from build123d import *

# Parameters (mm, degrees)
F0_W         = 50.8
F0_H         = 50.8
F16_DEPTH    = 0.635
F13_E4_W     = 50.8
F13_E4_H     = 25.4
F17_DEPTH    = 2.54
F11_E6_W     = 50.8
F11_E6_H     = 25.4
F11_E5_W     = 50.8
F11_E5_H     = 25.4
F18_DEPTH    = 2.54
F9_E0_W      = 25.4
F9_E0_H      = 25.4
F9_E3_W      = 25.4
F9_E3_H      = 25.4
F19_DEPTH    = 2.54
F7_E7_W      = 50.8
F7_E7_H      = 25.4
F20_DEPTH    = 2.54
F3_E1_W      = 50.8
F3_E1_H      = 25.4
F21_DEPTH    = 2.54
F1_E2_W      = 50.8
F1_E2_H      = 25.4
F22_DEPTH    = 2.54
F23_R        = 5.08
F24_T1_DEPTH = 51.7877054869


# Not quite as in the source:
# - a fillet or chamfer that OpenCascade refuses, or shapes differently, is made with other operations: its cross-section is extruded or revolved along the edge and cut away or added
# - the program builds the solid bodies; features that only make, move or delete a surface that nothing else refers to are left out


with BuildPart() as f16:
    # F0 (on Top) → F16 (new body)
    with BuildSketch(Plane.XY):
        Polygon((-25.4, 0), (0, 0), (25.4, 0), (25.4, 50.8), (-25.4, 50.8), align=None)
        Polygon((25.4, 0), (0, 0), (-25.4, 0), (-25.4, -50.8), (25.4, -50.8), align=None)
        with Locations((50.8, -25.4)):
            Rectangle(F0_W, F0_H)
        with Locations((50.8, 25.4)):
            Rectangle(F0_W, F0_H)
        with Locations((-50.8, -25.4)):
            Rectangle(F0_W, F0_H)
        with Locations((-50.8, 25.4)):
            Rectangle(F0_W, F0_H)
    extrude(amount=-F16_DEPTH)

    # F13_E4 (on explicit) → F17 (join, symmetric)
    with BuildSketch(Plane(origin=(-25.4, 0, 0), x_dir=(-1, 0, 0), z_dir=(0, 1, 0))):
        with Locations((25.4, 12.7)):
            Rectangle(F13_E4_W, F13_E4_H)
    extrude(amount=F17_DEPTH, both=True)

    # F11_E6 (on explicit) + F11_E5 (on explicit) → F18 (join, symmetric)
    with BuildSketch(Plane.YZ.offset(-25.4)):
        with Locations((25.4, 12.7)):
            Rectangle(F11_E6_W, F11_E6_H)
    with BuildSketch(Plane(origin=(-25.4, 0, 0), x_dir=(0, -1, 0), z_dir=(-1, 0, 0))):
        with Locations((25.4, 12.7)):
            Rectangle(F11_E5_W, F11_E5_H)
    extrude(amount=F18_DEPTH, both=True, dir=(1, 0, 0))

    # F9_E0 (on explicit) + F9_E3 (on explicit) → F19 (join, symmetric)
    with BuildSketch(Plane.XZ):
        with Locations((12.7, 12.7)):
            Rectangle(F9_E0_W, F9_E0_H)
    with BuildSketch(Plane(origin=(0, 0, 0), x_dir=(-1, 0, 0), z_dir=(0, 1, 0))):
        with Locations((12.7, 12.7)):
            Rectangle(F9_E3_W, F9_E3_H)
    extrude(amount=F19_DEPTH, both=True, dir=(0, -1, 0))

    # F7_E7 (on explicit) → F20 (join, symmetric)
    with BuildSketch(Plane.YZ.offset(25.4)):
        with Locations((25.4, 12.7)):
            Rectangle(F7_E7_W, F7_E7_H)
    extrude(amount=F20_DEPTH, both=True)

    # F3_E1 (on explicit) → F21 (join, symmetric)
    with BuildSketch(Plane(origin=(25.4, 0, 0), x_dir=(0, -1, 0), z_dir=(-1, 0, 0))):
        with Locations((25.4, 12.7)):
            Rectangle(F3_E1_W, F3_E1_H)
    extrude(amount=F21_DEPTH, both=True)

    # F1_E2 (on explicit) → F22 (join, symmetric)
    with BuildSketch(Plane(origin=(25.4, 0, 0), x_dir=(1, 0, 0), z_dir=(0, -1, 0))):
        with Locations((25.4, 12.7)):
            Rectangle(F1_E2_W, F1_E2_H)
    extrude(amount=F22_DEPTH, both=True)

    # F23
    f23_edges = [f16.edges().sort_by_distance(p)[0] for p in [
        (76.2, 0, -0.635),
    ]]
    fillet(f23_edges, radius=F23_R)

    # F24: fillet of radius 5.08 on 1 edges, made by hand

    # F24_s2 → F24_t1 (cut)
    with BuildSketch(Plane.YZ.offset(27.94)):
        with BuildLine():
            ThreePointArc((-50.8, -0.635), (-49.6106555752, -0.1613111503), (-48.3406555752, 0))
            Line((-48.3406555752, 0), (-50.8, 0))
            Line((-50.8, 0), (-50.8, -0.635))
        make_face()
    extrude(amount=F24_T1_DEPTH, mode=Mode.SUBTRACT)


solid = f16.part
Build history of the part. All positions in model axes, mm. A direction names the side the tool comes from. Give positions to 0.01 mm unless a question says otherwise; leave off trailing zeros. Loops run counter-clockwise (first coordinate to the right, second up) from the corner with the lowest first, then second, coordinate; pieces in that order, holes last. Notation, with made-up numbers: (20.5, 36.5) -> (38.5, 36.5) arc R32 cw to (38.5, 72.5) -> close; hole circle Ø7 at (75.25, -3). An arc over 180 degrees is marked (long way). Answer in a Markdown table with one row per item.
Item 1: Slice it at C-C on y = -29.5. Write the cut outline in (x, z) (3 decimals), plus the area to 3 significant figures.
Findings below:
| item | result |
|---|---|
| outline | (-76.2, -0.635) -> (71.12, -0.635) arc R5.08 ccw to (73.579, 0) -> (27.94, 0) -> (27.94, 25.4) -> (22.86, 25.4) -> (22.86, 0) -> (-22.86, 0) -> (-22.86, 25.4) -> (-27.94, 25.4) -> (-27.94, 0) -> (-76.2, 0) -> close |
| area | 353 mm² |
Item 2: Probe line 1 along X through (y, z) = (-25, 7.5); line 2 along Z through (x, y) = (29, 29.5) (3 decimals); line 3 along Y through (x, z) = (-67.5, 11.5). List the from-to ranges inside material, lowest first. Write a range as [from, to].
Findings below:
| item | result |
|---|---|
| line 1 | x = [-27.94, -22.86], [22.86, 27.94] |
| line 2 | z = [-0.635, 0] |
| line 3 | y = [-2.54, 2.54] |
Item 3: Flat gauge pins, fed straight in: P1, Ø3, axis at x = 5, z = 16.5, coming from the +Y side; P2, Ø4, axis at x = -10.5, z = 14.5, coming from the -Y side; P3, Ø8, axis at y = -33.5, z = 6.5, coming from the +X side. Where does each tip first touch, or does it go through?
Findings below:
| item | result |
|---|---|
| P1 | stops at y = 2.54 |
| P2 | stops at y = -2.54 |
| P3 | stops at x = 27.94 |
Item 4: Slice it at D-D on x = -16.5. Write the cut outline in (y, z) (3 decimals).
Findings below:
| item | result |
|---|---|
| outline | (-50.8, -0.635) -> (50.8, -0.635) -> (50.8, 0) -> (2.54, 0) -> (2.54, 25.4) -> (-2.54, 25.4) -> (-2.54, 0) -> (-50.8, 0) -> close |
Item 5: Slice it at A-A on x = 31.5. Write the cut outline in (y, z) (3 decimals).
Findings below:
| item | result |
|---|---|
| outline | (-50.8, -0.635) -> (50.8, -0.635) -> (50.8, 0) -> (2.54, 0) -> (2.54, 25.4) -> (-2.54, 25.4) -> (-2.54, 0) -> (-48.341, 0) arc R5.08 ccw to start |
Item 6: Slice it at B-B on z = 12.25. Write the cut outline in (x, y).
Findings below:
| item | result |
|---|---|
| outline | (-76.2, -2.54) -> (-27.94, -2.54) -> (-27.94, -50.8) -> (-22.86, -50.8) -> (-22.86, -2.54) -> (22.86, -2.54) -> (22.86, -50.8) -> (27.94, -50.8) -> (27.94, -2.54) -> (76.2, -2.54) -> (76.2, 2.54) -> (27.94, 2.54) -> (27.94, 50.8) -> (22.86, 50.8) -> (22.86, 2.54) -> (-22.86, 2.54) -> (-22.86, 50.8) -> (-27.94, 50.8) -> (-27.94, 2.54) -> (-76.2, 2.54) -> close |
Item 7: Tool access for faces 4 (the flat face through (-52, -26, 0)), 5 (the flat face through (22.86, 26, 13)), 6 (the flat face through (52, 2.54, 13)), 7 (the flat face through (0, -2.54, 13)): list every direction of +Z, -Z, +X, -X, +Y, -Y with a clear straight run to the whole face (end or side of a thin tool).
Findings below:
| item | result |
|---|---|
| face 4 | +Z, -X, -Y |
| face 5 | +Z, +Y |
| face 6 | +Z, +X, +Y |
| face 7 | +Z, -Y |
Item 8: Mould opens along X. For faces 1 (the flat face through (-27.94, 27, 13)), 2 (the flat face through (0, 27, 0)), 3 (the flat face through (-52, 2.54, 13)) say: pulls with the +X half, pulls with the -X half, needs draft (parallel to the pull), parting line crosses it, or undercut.
Findings below:
| item | result |
|---|---|
| face 1 | pulls with the -X half |
| face 2 | undercut |
| face 3 | needs draft |
